```python
from build123d import *

# Parameters (mm, degrees)
ESQUISSE1_W             = 596.9
ESQUISSE1_H             = 21.59
BOSS_EXTRU_1_DEPTH      = 3.175
ESQUISSE4_W             = 74.8125
ESQUISSE4_H             = 3.18
ESQUISSE4_H_2           = 3.175
ESQUISSE4_W_2           = 37.40625
ENL_V_MAT_EXTRU_3_DEPTH = 299.662041696
ESQUISSE5_R             = 4.7244
ESQUISSE5_W             = 6.858
ESQUISSE5_H             = 6.35
ENL_V_MAT_EXTRU_4_DEPTH = 299.662041696


with BuildPart() as part:
    # Esquisse1 → Boss.-Extru.1 (new body)
    with BuildSketch(Plane.XY):
        Rectangle(ESQUISSE1_W, ESQUISSE1_H)
    extrude(amount=BOSS_EXTRU_1_DEPTH)

    # Esquisse4 → Enlèv. mat.-Extru.3 (cut, through all)
    with BuildSketch(Plane.XY.offset(3.175)):
        with Locations((0, 9.205)):
            Rectangle(ESQUISSE4_W, ESQUISSE4_H)
        with Locations((-149.225, 9.2075)):
            Rectangle(ESQUISSE4_W, ESQUISSE4_H_2)
        with Locations((-279.746875, 9.2075)):
            Rectangle(ESQUISSE4_W_2, ESQUISSE4_H_2)
        with Locations((279.746875, 9.2075)):
            Rectangle(ESQUISSE4_W_2, ESQUISSE4_H_2)
        with Locations((149.225, 9.2075)):
            Rectangle(ESQUISSE4_W, ESQUISSE4_H_2)
    enl_v_mat_extru_3 = extrude(amount=-ENL_V_MAT_EXTRU_3_DEPTH, mode=Mode.SUBTRACT)

    # Symétrie3: Enlèv. mat.-Extru.3 across plane
    add(enl_v_mat_extru_3.mirror(Plane.ZX), mode=Mode.SUBTRACT)

    # Esquisse5 → Enlèv. mat.-Extru.4 (cut, through all)
    with BuildSketch(Plane.XY.offset(3.175)):
        with Locations((-266.7, 0)):
            Circle(ESQUISSE5_R)
        with Locations((-244.475, 0)):
            Rectangle(ESQUISSE5_W, ESQUISSE5_H)
        with Locations((-288.925, 0)):
            Rectangle(ESQUISSE5_W, ESQUISSE5_H)
    enl_v_mat_extru_4 = extrude(amount=-ENL_V_MAT_EXTRU_4_DEPTH, mode=Mode.SUBTRACT)

    # Symétrie4: Enlèv. mat.-Extru.4 across plane
    add(enl_v_mat_extru_4.mirror(Plane(origin=(0, 0, 0), x_dir=(0, 0, 1), z_dir=(1, 0, 0))), mode=Mode.SUBTRACT)


solid = part.part
```
Can you work these out from the model? Positions are in its coordinate system, mm. Coordinates: 2 decimals unless noted, no trailing zeros. Write each loop counter-clockwise with the first axis right and the second up, starting at its lowest first coordinate (ties: lowest second). Pieces come first, ordered by that corner, then holes. Notation, with made-up numbers: (54, -37) - (96, -37) arc R20 cw to (96, -10) - close; hole circle Ø5 at (6, 10). An arc over 180 degrees is marked (long way). Return JSON: item names as keys, results as strings.
Q1. If we section it at B-B (x = -154): Please give me the cut outline in (y, z) (3 decimals), then the cut area to 3 significant figures.
Computed values:
{"outline": "(-7.62, 0) - (7.62, 0) - (7.62, 3.175) - (-7.62, 3.175) - close", "area": "48.4 mm2"}
Q2. Please list where these lines run through material, in increasing order: L1, parallel to X at y = 8.5, z = 0.95; L2, parallel to Y at x = 266.7, z = 1.2; L3, parallel to Y at x = -273, z = 0.1. Write a range as from..to.
Computed values:
{"L1": "x = -261.04..-186.63, -111.82..-37.41, 37.41..111.82, 186.63..261.04", "L2": "y = -7.62..-4.72, 4.72..7.62", "L3": "y = -7.62..7.62"}
Q3. Thinking about a two-plate mould opening in X: for faces 1 (the cylindrical face through (262.194, 1.419, 1.61)), 2 (the flat face through (-4, 0, 0)), 3 (the cylindrical face through (-262.194, 1.419, 1.61)), which applies, +X half, -X half, draft (parallel to the pull), parting line (faces both ways), or undercut?
Computed values:
{"face 1": "undercut", "face 2": "draft", "face 3": "undercut"}
Q4. If we section it at A-A (z = 0.9): Count the separate pieces of the cut face and the enclosed holes in it, then the cut area to 3 significant figures.
Computed values:
{"separate pieces": "1", "enclosed holes": "6", "area": "10,700 mm2"}
Q5. I'm going to push flat-ended pins straight in: pin 1 Ø1 at (x, z) = (-10, 1) entering from -Y (3 decimals); pin 2 Ø1 at (x, z) = (176.5, 1) entering from +Y. Where does each tip first touch, or does it pass through?
Computed values:
{"pin 1": "stops at y = -7.615", "pin 2": "stops at y = 7.62"}
